The drawing under review shows one solid part. Ordinate dimensions are in mm from its lowest x, y, z. Give positions to 0.01 mm unless a question says otherwise; leave off trailing zeros. Loops run counter-clockwise (first coordinate to the right, second up) from the corner with the lowest first, then second, coordinate; pieces in that order, holes last. Notation, with made-up numbers: (-5.5, 8.5) - (19.5, 8.5) arc R27 cw to (19.5, 31.5) - close; hole circle Ø3 at (-3.5, 72). An arc over 180 degrees is marked (long way). Answer as CSV lines item,"result".
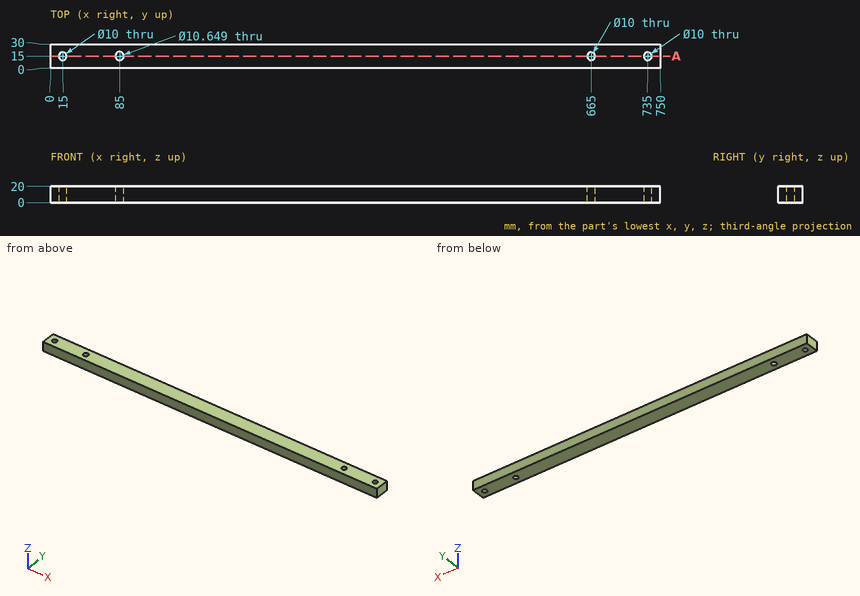
1) Wall thickness on line 1 (Y direction, x = 85, z = 14.5) (1 decimal); line 2 (X direction, y = 12.5, z = 10.25); line 3 (X direction, y = 13.25, z = 5.5) (1 decimal): over which ranges is each line inside the solid? List them lowest first. Write a range as from..to.
From the geometry:
line 1,"y = 0..9.7, 20.3..30"
line 2,"x = 0..10.67, 19.33..80.3, 89.7..660.67, 669.33..730.67, 739.33..750"
line 3,"x = 0..10.3, 19.7..80, 90..660.3, 669.7..730.3, 739.7..750"
2) Consider section A-A on y = 15. Write out the cut boundary in (x, z) (1 decimal).
From the geometry:
outline,"(0, 0) - (10, 0) - (10, 20) - (0, 20) - close; (20, 0) - (79.7, 0) - (79.7, 20) - (20, 20) - close; (90.3, 0) - (660, 0) - (660, 20) - (90.3, 20) - close; (670, 0) - (730, 0) - (730, 20) - (670, 20) - close; (740, 0) - (750, 0) - (750, 20) - (740, 20) - close"
3) Insertion check: P1, Ø6, axis at x = 735, y = 15, coming from the +Z side. The pin has a flat end and moves straight along its axis. Give the tip position at first contact, or say it passes through.
From the geometry:
P1,"passes through"
